Source: CAD feature listing. Evaluate the final solid. Frame: model axes, mm. Face numbers are marked on the shaded views. A direction names the side the tool comes from. Coordinates: 2 decimals unless noted, no trailing zeros. Loops run counter-clockwise (first coordinate to the right, second up) from the corner with the lowest first, then second, coordinate; pieces in that order, holes last. Notation, with made-up numbers: (-27, 44) -> (9, 44) arc R32 cw to (9, 70) -> close; hole circle Ø11 at (53.5, 84). An arc over 180 degrees is marked (long way). Answer as a JSON object with one key per item and string values. Group by question number.
from build123d import *

# Parameters (mm, degrees)
SKETCH1_W                 = 31
SKETCH1_H                 = 12
BOSS_EXTRUDE1_DEPTH       = 5
SHELL1_T                  = -2.6
SHELL1_THICKNESS_2_FACE_W = 6.8
SHELL1_THICKNESS_2_FACE_H = 25.8
SHELL1_THICKNESS_2_DEPTH  = 1.1
SKETCH2_W                 = 12
SKETCH2_H                 = 12
CUT_EXTRUDE1_DEPTH        = 2
FILLET1_R                 = 2
FILLET2_R                 = 1


with BuildPart() as part:
    # Sketch1 → Boss-Extrude1 (new body)
    with BuildSketch(Plane(origin=(0, 0, 0), x_dir=(1, 0, 0), z_dir=(0, 1, 0))):
        Rectangle(SKETCH1_W, SKETCH1_H)
    extrude(amount=BOSS_EXTRUDE1_DEPTH)

    # Shell1
    shell1_openings = [part.faces().sort_by_distance(p)[0] for p in [
        (0, 5, 0),
    ]]
    offset(amount=SHELL1_T, openings=shell1_openings, kind=Kind.INTERSECTION)

    # Shell1 thickness 2 face (on inner face of the shell) → Shell1 thickness 2 (cut)
    with BuildSketch(Plane(origin=(0, 2.6, 0), x_dir=(0, 0, -1), z_dir=(0, -1, 0))):
        Rectangle(SHELL1_THICKNESS_2_FACE_W, SHELL1_THICKNESS_2_FACE_H)
    extrude(amount=SHELL1_THICKNESS_2_DEPTH, mode=Mode.SUBTRACT)

    # Sketch2 → Cut-Extrude1 (cut)
    with BuildSketch(Plane(origin=(0, 5, 0), x_dir=(1, 0, 0), z_dir=(0, 1, 0))):
        Rectangle(SKETCH2_W, SKETCH2_H)
    extrude(amount=-CUT_EXTRUDE1_DEPTH, mode=Mode.SUBTRACT)

    # Fillet1
    fillet1_edges = [part.edges().sort_by_distance(p)[0] for p in [
        (15.5, 2.5, 6),
        (-15.5, 2.5, 6),
        (-15.5, 2.5, -6),
        (15.5, 2.5, -6),
    ]]
    fillet(fillet1_edges, radius=FILLET1_R)

    # Fillet2
    fillet2_edges = [part.edges().sort_by_distance(p)[0] for p in [
        (12.9, 3.25, 3.4),
        (12.9, 3.25, -3.4),
        (-12.9, 3.25, -3.4),
        (-12.9, 3.25, 3.4),
    ]]
    fillet(fillet2_edges, radius=FILLET2_R)


solid = part.part
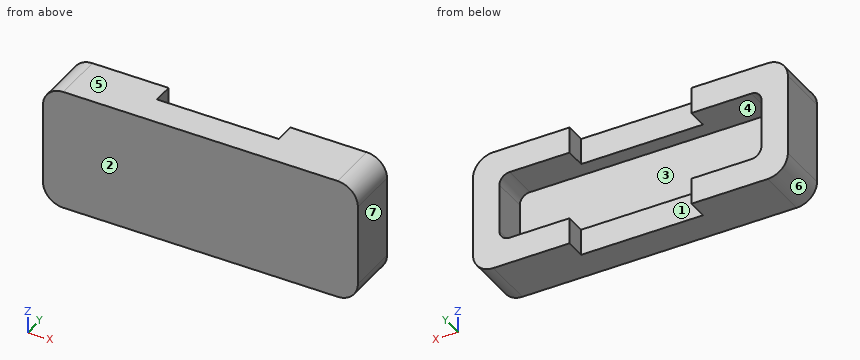
1. Section query C-C on x = 7. Return loops of the section in (y, z), then the cut area to 3 significant figures.
2. Pin query (flat end, axial travel): pin 1 Ø2 at (y, z) = (4.5, 4.5) entering from -X; pin 2 Ø2 at (x, z) = (-2.5, -5) entering from +Y; pin 3 Ø2 at (x, z) = (1.5, -0.5) entering from +Y. Return the tip coordinate at first contact, or that it passes through.
3. Mould query, pull axis Z, two halves, no side actions, for the marked faces 4, 5, 6 and 7. Classes: pulls with the +Z half, pulls with the -Z half, needs draft (parallel to the pull), parting line crosses it, or undercut.
4. Reachability of the marked faces 1, 2 and 3 from +Z, -Z, +X, -X, +Y, -Y: full face, straight path, thin tool, end or side. Return the list, or none.
5. Section query D-D on y = 2.2. Return loops of the section in (x, z).
6. Section query A-A on y = 4. Return loops of the section in (x, z), then the cut area to 3 significant figures.
7. Ray query, L1, parallel to X at y = 2.5, z = -0.25; L2, parallel to Z at x = -5.5, y = 2.6; L3, parallel to X at y = 4.35, z = 4. Return the intervals inside material, ascending.
8. Section query B-B on z = 3. Return loops of the section in (x, y), then the cut area to 3 significant figures.
Solved:
{
 "1": {"outline": "(0, -6) -> (5, -6) -> (5, -3.4) -> (1.5, -3.4) -> (1.5, 3.4) -> (5, 3.4) -> (5, 6) -> (0, 6) -> close", "area": "36.2 mm^2"},
 "2": {"pin 1": "x = -15.5", "pin 2": "y = 3", "pin 3": "y = 1.5"},
 "3": {"face 4": "undercut", "face 5": "pulls with the +Z half", "face 6": "pulls with the -Z half", "face 7": "needs draft"},
 "4": {"face 1": "+Z, -Z, +Y", "face 2": "+Z, -Z, +X, -X, -Y", "face 3": "+Y"},
 "5": {"outline": "(-15.5, -4) arc R2 ccw to (-13.5, -6) -> (13.5, -6) arc R2 ccw to (15.5, -4) -> (15.5, 4) arc R2 ccw to (13.5, 6) -> (-13.5, 6) arc R2 ccw to (-15.5, 4) -> close; hole (-12.9, -2.4) arc R1 ccw to (-11.9, -3.4) -> (11.9, -3.4) arc R1 ccw to (12.9, -2.4) -> (12.9, 2.4) arc R1 ccw to (11.9, 3.4) -> (-11.9, 3.4) arc R1 ccw to (-12.9, 2.4) -> close"},
 "6": {"outline": "(-15.5, -4) arc R2 ccw to (-13.5, -6) -> (-6, -6) -> (-6, -3.4) -> (-11.9, -3.4) arc R1 cw to (-12.9, -2.4) -> (-12.9, 2.4) arc R1 cw to (-11.9, 3.4) -> (-6, 3.4) -> (-6, 6) -> (-13.5, 6) arc R2 ccw to (-15.5, 4) -> close; (6, -6) -> (13.5, -6) arc R2 ccw to (15.5, -4) -> (15.5, 4) arc R2 ccw to (13.5, 6) -> (6, 6) -> (6, 3.4) -> (11.9, 3.4) arc R1 cw to (12.9, 2.4) -> (12.9, -2.4) arc R1 cw to (11.9, -3.4) -> (6, -3.4) -> close", "area": "132 mm^2"},
 "7": {"L1": "-15.5 to -12.9, 12.9 to 15.5", "L2": "-6 to -3.4, 3.4 to 6", "L3": "-15.5 to -6, 6 to 15.5"},
 "8": {"outline": "(-15.5, 0) -> (15.5, 0) -> (15.5, 5) -> (12.7, 5) -> (12.7, 1.5) -> (-12.7, 1.5) -> (-12.7, 5) -> (-15.5, 5) -> close", "area": "66.1 mm^2"}
}
